```python
from build123d import *
from build123d.topology import SkipClean

# Parameters (mm, degrees)
SKETCH1_W               = 110
SKETCH1_H               = 110
BOSS_EXTRUDE1_DEPTH     = 10
CUT_EXTRUDE1_DEPTH      = 1
CUT_EXTRUDE1_DEPTH_BACK = 2.5
SKETCH2_W               = 105
SKETCH2_H               = 105
SKETCH5_R               = 2.75
CUT_EXTRUDE2_DEPTH      = 10
SKETCH6_R               = 3.5
CUT_EXTRUDE3_DEPTH      = 12.5
BOSS_EXTRUDE2_START     = 5
BOSS_EXTRUDE2_DEPTH     = 5
BOSS_EXTRUDE3_START     = 5
BOSS_EXTRUDE3_DEPTH     = 5
CUT_EXTRUDE5_START      = -5
SKETCH20_R              = 6
SKETCH20_R_2            = 3.5
CUT_EXTRUDE5_DEPTH      = 5
FILLET1_R               = 0.8
SKETCH23_R              = 3
CUT_EXTRUDE6_DEPTH      = 10


with BuildPart() as part:
    # Sketch1 → Boss-Extrude1 (new body)
    with BuildSketch(Plane(origin=(0, 0, 0), x_dir=(1, 0, 0), z_dir=(0, 1, 0))):
        with Locations((7.264150943, -17.018867925)):
            Rectangle(SKETCH1_W, SKETCH1_H)
    extrude(amount=BOSS_EXTRUDE1_DEPTH)

    # Sketch2 → Cut-Extrude1 (cut, two sides: drawn at the far end of the back side and taken through both)
    with BuildSketch(Plane(origin=(0, 10, 0), x_dir=(1, 0, 0), z_dir=(0, 1, 0)).offset(-CUT_EXTRUDE1_DEPTH_BACK)):
        with Locations((7.264150943, -17.018867925)):
            Rectangle(SKETCH2_W, SKETCH2_H)
    extrude(amount=CUT_EXTRUDE1_DEPTH + CUT_EXTRUDE1_DEPTH_BACK, mode=Mode.SUBTRACT)

    # Sketch5 → Cut-Extrude2 (cut)
    with BuildSketch(Plane(origin=(0, 7.5, 0), x_dir=(1, 0, 0), z_dir=(0, 1, 0))):
        with Locations(Location((-3.235849057, 11.481132075, 0), (0, 0, 270))):
            Circle(SKETCH5_R)
        with Locations(Location((17.764150943, 11.481132075, 0), (0, 0, 270))):
            Circle(SKETCH5_R)
        with Locations(Location((-3.235849057, -45.518867925, 0), (0, 0, 270))):
            Circle(SKETCH5_R)
        with Locations(Location((17.764150943, -45.518867925, 0), (0, 0, 270))):
            Circle(SKETCH5_R)
        with Locations(Location((-21.235849057, -6.518867925, 0), (0, 0, 270))):
            Circle(SKETCH5_R)
        with Locations(Location((-21.235849057, -27.518867925, 0), (0, 0, 270))):
            Circle(SKETCH5_R)
        with Locations(Location((35.764150943, -6.518867925, 0), (0, 0, 270))):
            Circle(SKETCH5_R)
        with Locations(Location((35.764150943, -27.518867925, 0), (0, 0, 270))):
            Circle(SKETCH5_R)
    extrude(amount=-CUT_EXTRUDE2_DEPTH, mode=Mode.SUBTRACT)

    # Sketch6 → Cut-Extrude3 (cut)
    with BuildSketch(Plane(origin=(0, 7.5, 0), x_dir=(1, 0, 0), z_dir=(0, 1, 0))):
        with Locations(Location((-10.235849057, 17.981132075, 0), (0, 0, 270))):
            Circle(SKETCH6_R)
        with Locations(Location((24.764150943, 17.981132075, 0), (0, 0, 270))):
            Circle(SKETCH6_R)
        with Locations(Location((-10.235849057, -52.018867925, 0), (0, 0, 270))):
            Circle(SKETCH6_R)
        with Locations(Location((24.764150943, -52.018867925, 0), (0, 0, 270))):
            Circle(SKETCH6_R)
    extrude(amount=-CUT_EXTRUDE3_DEPTH, mode=Mode.SUBTRACT)

    # Sketch8 → Boss-Extrude2 (add)
    with SkipClean():  # the faces are left unmerged after this step: merging them gives an invalid solid
        with BuildSketch(Plane(origin=(0, 7.5, 0), x_dir=(1, 0, 0), z_dir=(0, 1, 0)).offset(BOSS_EXTRUDE2_START)):
            with BuildLine():
                Line((19.507777717, 19.600322443), (21.41925455, 19.01150488))
                ThreePointArc((21.41925455, 19.01150488), (27.328928164, 20.362710923), (25.544270116, 14.569180423))
                Line((25.544270116, 14.569180423), (25.990077565, 12.619384146))
                ThreePointArc((25.990077565, 12.619384146), (28.794597548, 21.723689637), (19.507777717, 19.600322443))
            make_face()
        extrude(amount=-BOSS_EXTRUDE2_DEPTH)

    # Sketch15 → Boss-Extrude3 (add)
    with SkipClean():  # the faces are left unmerged after this step: merging them gives an invalid solid
        with BuildSketch(Plane(origin=(0, 7.5, 0), x_dir=(1, 0, 0), z_dir=(0, 1, 0)).offset(BOSS_EXTRUDE3_START)):
            with BuildLine():
                Line((-11.422433018, 12.791454335), (-11.01596823, 14.569180423))
                ThreePointArc((-11.01596823, 14.569180423), (-12.800626277, 20.362710923), (-6.890952663, 19.01150488))
                Line((-6.890952663, 19.01150488), (-5.148164315, 19.548359092))
                ThreePointArc((-5.148164315, 19.548359092), (-14.136949837, 21.6035828), (-11.422433018, 12.791454335))
            make_face()
            with BuildLine():
                Line((-11.461750614, -46.657229614), (-11.01596823, -48.606916272))
                ThreePointArc((-11.01596823, -48.606916272), (-12.800626277, -54.400446772), (-6.890952663, -53.049240729))
                Line((-6.890952663, -53.049240729), (-4.979583295, -53.638025188))
                ThreePointArc((-4.979583295, -53.638025188), (-14.266213261, -55.761348971), (-11.461750614, -46.657229614))
            make_face()
            with BuildLine():
                Line((19.507885182, -53.638025188), (21.41925455, -53.049240729))
                ThreePointArc((21.41925455, -53.049240729), (27.328928164, -54.400446772), (25.544270116, -48.606916272))
                Line((25.544270116, -48.606916272), (25.990052501, -46.657229614))
                ThreePointArc((25.990052501, -46.657229614), (28.794515147, -55.761348971), (19.507885182, -53.638025188))
            make_face()
        extrude(amount=-BOSS_EXTRUDE3_DEPTH)

    # Sketch20 → Cut-Extrude5 (cut)
    # profile 1 of 4: a face of its own
    with SkipClean():  # the faces are left unmerged after this step: merging them gives an invalid solid
        with BuildSketch(Plane.XZ.offset(CUT_EXTRUDE5_START)):
            with Locations(Location((-10.235849057, 52.018867925, 0), (0, 0, 270))):
                Circle(SKETCH20_R)
            with Locations(Location((-10.235849057, 52.018867925, 0), (0, 0, 17.121096397))):
                Circle(SKETCH20_R_2, mode=Mode.SUBTRACT)
        # profile 2 of 4: a face of its own
        with BuildSketch(Plane.XZ.offset(CUT_EXTRUDE5_START)):
            with Locations(Location((-10.235849057, -17.981132075, 0), (0, 0, 270))):
                Circle(SKETCH20_R)
            with Locations(Location((-10.235849057, -17.981132075, 0), (0, 0, 102.878903603))):
                Circle(SKETCH20_R_2, mode=Mode.SUBTRACT)
        # profile 3 of 4: a face of its own
        with BuildSketch(Plane.XZ.offset(CUT_EXTRUDE5_START)):
            with Locations(Location((24.764150943, -17.981132075, 0), (0, 0, 270))):
                Circle(SKETCH20_R)
            with Locations(Location((24.764150943, -17.981132075, 0), (0, 0, 77.121096397))):
                Circle(SKETCH20_R_2, mode=Mode.SUBTRACT)
        # profile 4 of 4: a face of its own
        with BuildSketch(Plane.XZ.offset(CUT_EXTRUDE5_START)):
            with Locations(Location((24.764150943, 52.018867925, 0), (0, 0, 270))):
                Circle(SKETCH20_R)
            with Locations(Location((24.764150943, 52.018867925, 0), (0, 0, 162.878903603))):
                Circle(SKETCH20_R_2, mode=Mode.SUBTRACT)
        extrude(amount=CUT_EXTRUDE5_DEPTH, mode=Mode.SUBTRACT)

    # Fillet1
    fillet1_edges = [part.edges().sort_by_distance(p)[0] for p in [
        (62.264150943, 10, 17.018867925),
        (7.264150943, 10, -35.481132075),
        (59.764150943, 10, 17.018867925),
        (7.264150943, 10, 69.518867925),
        (-45.235849057, 10, 17.018867925),
        (7.264150943, 10, -37.981132075),
        (-47.735849057, 10, 17.018867925),
        (7.264150943, 0, -37.981132075),
        (62.264150943, 0, 17.018867925),
        (7.264150943, 0, 72.018867925),
        (-47.735849057, 0, 17.018867925),
        (-47.735849057, 5, -37.981132075),
        (62.264150943, 5, -37.981132075),
        (62.264150943, 5, 72.018867925),
        (-47.735849057, 5, 72.018867925),
        (7.264150943, 10, 72.018867925),
    ]]
    fillet(fillet1_edges, radius=FILLET1_R)

    # Sketch23 → Cut-Extrude6 (cut)
    with SkipClean():  # the faces are left unmerged after this step: merging them gives an invalid solid
        with BuildSketch(Plane(origin=(0, 7.5, 0), x_dir=(1, 0, 0), z_dir=(0, 1, 0))):
            with Locations(Location((52.264150943, 27.981132075, 0), (0, 0, 270))):
                Circle(SKETCH23_R)
        extrude(amount=-CUT_EXTRUDE6_DEPTH, mode=Mode.SUBTRACT)


solid = part.part
```
Input: part model. Units: mm. Frame: model coordinates. A direction names the side the tool comes from. Coordinates: 2 decimals unless noted, no trailing zeros. Loops run counter-clockwise (first coordinate to the right, second up) from the corner with the lowest first, then second, coordinate; pieces in that order, holes last. Notation, with made-up numbers: (-10.5, -18) -> (4.5, -18) arc R35 ccw to (4.5, 14) -> close; hole circle Ø5 at (14.25, 60.5). An arc over 180 degrees is marked (long way). Use a Markdown table: item, result.
1) Cut plane B-B (z = 14.5). Return the cut outline in (x, y), then the cut area to 3 significant figures.
Results found:
| item | result |
|---|---|
| outline | (-47.74, 0.8) arc R0.8 ccw to (-46.94, 0) -> (61.46, 0) arc R0.8 ccw to (62.26, 0.8) -> (62.26, 9.2) arc R0.8 ccw to (61.46, 10) -> (60.56, 10) arc R0.8 ccw to (59.76, 9.2) -> (59.76, 7.5) -> (-45.24, 7.5) -> (-45.24, 9.2) arc R0.8 ccw to (-46.04, 10) -> (-46.94, 10) arc R0.8 ccw to (-47.74, 9.2) -> close |
| area | 837 mm2 |
2) Pull-direction query (Z, two-part tool) for faces 1 (the cylindrical face through (38.49, 3.8, 6.16)), 2 (the flat face through (7, 5, -37.981)), 3 (the flat face through (-47.736, 5, 18)), 4 (the cylindrical face through (55.24, 3.8, -28.37)); classes: released by +Z, released by -Z, zero draft, split by the parting line, or undercut.
Results found:
| item | result |
|---|---|
| face 1 | undercut |
| face 2 | released by -Z |
| face 3 | zero draft |
| face 4 | undercut |
3) Cut plane A-A (y = 2.75). Give the number of separate pieces and of enclosed holes in the cut face, then the cut area to 3 significant figures.
Results found:
| item | result |
|---|---|
| separate pieces | 1 |
| enclosed holes | 13 |
| area | 11,400 mm2 |
4) Contact query for flat-ended pins moving along their axis: pin 1 (3.5 mm diameter, centred on x = -21.24, z = 27.52, fed in from -Y); pin 2 (9 mm diameter, centred on x = 24.76, z = -17.98, fed in from -Y); pin 3 (11 mm diameter, centred on x = -10.24, z = -17.98, fed in from +Y); pin 4 (6.5 mm diameter, centred on x = -3.24, z = -11.48, fed in from +Y). Output: stop coordinate, or through.
Results found:
| item | result |
|---|---|
| pin 1 | passes through |
| pin 2 | stops at y = 5 |
| pin 3 | stops at y = 12.5 |
| pin 4 | stops at y = 7.5 |
5) Access query for faces 5 (the flat face through (-13, 5, -21)), 6 (the cylindrical face through (28.903, 10.035, -21.604)), 7 (the flat face through (62.264, 5, 18)). Directions: +Z, -Z, +X, -X, +Y, -Y. A direction counts if a zero-diameter tool reaches every point of the face in a straight line with its end or side. Return the directions, or none.
Results found:
| item | result |
|---|---|
| face 5 | -Y |
| face 6 | +Y |
| face 7 | +Z, -Z, +X, +Y, -Y |
6) Material intervals for line 1 along Z through (x, y) = (-3.5, 6.75); line 2 along X through (y, z) = (6, -11.5); line 3 along Z through (x, y) = (49.5, 8.25), sorted ascending. Write a range as from..to.
Results found:
| item | result |
|---|---|
| line 1 | z = -37.98..-14.22, -8.74..42.78, 48.26..72.02 |
| line 2 | x = -47.74..-5.99, -0.49..15.01, 20.51..62.26 |
| line 3 | z = -37.98..-35.48, 69.52..72.02 |
